Design review of the part built by this model. Coordinates are the model's own, in mm. Face numbers are marked on the shaded views. A direction names the side the tool comes from. Coordinates: 2 decimals unless noted, no trailing zeros. Write each loop counter-clockwise with the first axis right and the second up, starting at its lowest first coordinate (ties: lowest second). Pieces come first, ordered by that corner, then holes. Notation, with made-up numbers: M 72,20.5 L 76,20.5 A18 ccw 76,31.5 Z; hole C 67,-22 d1. An arc over 180 degrees is marked long. Write item = value, one per line.
```python
from build123d import *

# Parameters (mm, degrees)
BOSS_EXTRUDE1_DEPTH = 24
SKETCH1_4_W         = 12
SKETCH1_4_H         = 25
BOSS_EXTRUDE3_DEPTH = 60
BOSS_EXTRUDE5_DEPTH = 80
CUT_EXTRUDE4_DEPTH  = 104
BOSS_EXTRUDE6_DEPTH = 46
SKETCH5_W           = 44
SKETCH5_H           = 20
CUT_EXTRUDE5_DEPTH  = 46


with BuildPart() as part:
    # Sketch1 → Boss-Extrude1 (new body)
    with BuildSketch(Plane(origin=(0, 0, 0), x_dir=(1, 0, 0), z_dir=(0, 1, 0))):
        with BuildLine():
            Line((-50.214859888, 8.694484644), (-50.214859888, -16.305515356))
            Line((-50.214859888, -16.305515356), (-42.214859888, -16.305515356))
            ThreePointArc((-42.214859888, -16.305515356), (-12.214859888, 13.694484644), (17.785140112, -16.305515356))
            Line((17.785140112, -16.305515356), (25.785140112, -16.305515356))
            Line((25.785140112, -16.305515356), (25.785140112, 8.694484644))
            Line((25.785140112, 8.694484644), (25.785140112, 16.694484644))
            Line((25.785140112, 16.694484644), (-50.214859888, 16.694484644))
            Line((-50.214859888, 16.694484644), (-50.214859888, 8.694484644))
        make_face()
    extrude(amount=BOSS_EXTRUDE1_DEPTH)

    # Sketch1<4> → Boss-Extrude3 (add)
    with BuildSketch(Plane(origin=(0, 0, 0), x_dir=(1, 0, 0), z_dir=(0, 1, 0))):
        with Locations((-56.214859888, -3.805515356)):
            Rectangle(SKETCH1_4_W, SKETCH1_4_H)
        with Locations((31.785140112, -3.805515356)):
            Rectangle(SKETCH1_4_W, SKETCH1_4_H)
    extrude(amount=BOSS_EXTRUDE3_DEPTH)

    # Sketch1<7> → Boss-Extrude5 (add)
    with BuildSketch(Plane(origin=(0, 0, 0), x_dir=(1, 0, 0), z_dir=(0, 1, 0))):
        Polygon((-62.214859888, 28.694484644), (-62.214859888, 8.694484644), (-50.214859888, 8.694484644), (-50.214859888, 16.694484644), (25.785140112, 16.694484644), (25.785140112, 8.694484644), (37.785140112, 8.694484644), (37.785140112, 28.694484644), align=None)
    extrude(amount=BOSS_EXTRUDE5_DEPTH)

    # Sketch3 → Cut-Extrude4 (cut)
    with BuildSketch(Plane.ZY.offset(62.214859888)):
        Polygon((16.305515356, 24), (-8.694484644, 60), (16.305515356, 60), align=None)
    extrude(amount=-CUT_EXTRUDE4_DEPTH, mode=Mode.SUBTRACT)

    # Sketch1<8> → Boss-Extrude6 (add)
    with BuildSketch(Plane(origin=(0, 0, 0), x_dir=(1, 0, 0), z_dir=(0, 1, 0))):
        with BuildLine():
            ThreePointArc((17.785140112, -16.305515356), (-12.214859888, 13.694484644), (-42.214859888, -16.305515356))
            Line((-42.214859888, -16.305515356), (-30.214859888, -16.305515356))
            ThreePointArc((-30.214859888, -16.305515356), (-12.214859888, 1.694484644), (5.785140112, -16.305515356))
            Line((5.785140112, -16.305515356), (17.785140112, -16.305515356))
        make_face()
    extrude(amount=BOSS_EXTRUDE6_DEPTH)

    # Sketch5 → Cut-Extrude5 (cut)
    with BuildSketch(Plane.XY.offset(-16.694484644)):
        with Locations((-12.214859888, 58)):
            Rectangle(SKETCH5_W, SKETCH5_H)
    extrude(amount=-CUT_EXTRUDE5_DEPTH, mode=Mode.SUBTRACT)


solid = part.part
```
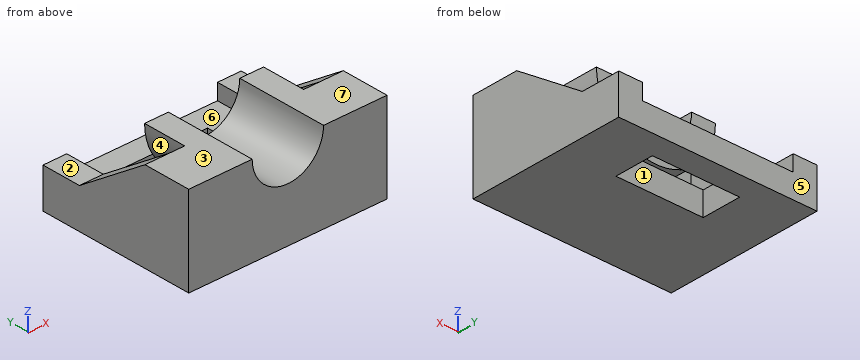
Q1. Consider section B-B, the plane z = 1.5. State the section outline as (x, y) points, and give its area (3 significant figures).
Check result:
outline = M -62.21,0 L -22.45,0 L -22.45,46 L -38.31,46 L -38.31,24 L -50.21,24 L -50.21,45.32 L -62.21,45.32 Z; M -1.98,0 L 37.79,0 L 37.79,45.32 L 25.79,45.32 L 25.79,24 L 13.88,24 L 13.88,46 L -1.98,46 Z
area = 3,120 mm²
Q2. For P1, Ø24, axis at x = -15, z = 7, coming from the +Y side; P2, Ø4, axis at x = -44, z = 8.5, coming from the +Y side; P3, Ø9.5, axis at x = -59, y = 67.5, coming from the +Z side, all flat-tipped, find the tip position at first contact; note any pin that passes through.
Check result:
P1 = 46
P2 = 24
P3 = -8.69
Q3. Consider section A-A, the plane y = 65. State the section outline as (x, z) points, and give its area (3 significant figures).
Check result:
outline = M -62.21,-28.69 L -34.21,-28.69 L -34.21,-16.69 L -50.21,-16.69 L -50.21,-8.69 L -62.21,-8.69 Z; M 9.79,-28.69 L 37.79,-28.69 L 37.79,-8.69 L 25.79,-8.69 L 25.79,-16.69 L 9.79,-16.69 Z
area = 864 mm²
Q4. Machinability: for the marked faces 1, 2, 3 and 4, which of the approach directions +Z, -Z, +X, -X, +Y, -Y give a long, thin tool a straight path to every point of the face, cutting with its end or side? Answer none if there is none.
Check result:
face_1 = +Z, -Z
face_2 = +Z, +X, -X, +Y
face_3 = +Z, +X, -X, +Y, -Y
face_4 = +Y
Q5. Consider section C-C, the plane x = -27. State the section outline as (y, z) points.
Check result:
outline = M 0,-28.69 L 48,-28.69 L 48,-16.69 L 24,-16.69 L 24,-9.8 L 46,-9.8 L 46,6.04 L 0,6.04 Z; M 68,-28.69 L 80,-28.69 L 80,-16.69 L 68,-16.69 Z
Q6. Consider section D-D, the plane z = -25. State the section outline as (x, y) points.
Check result:
outline = M -62.21,0 L 37.79,0 L 37.79,80 L -62.21,80 Z; hole M -34.21,48 L 9.79,48 L 9.79,68 L -34.21,68 Z
Q7. Wall thickness on line 1 (X direction, y = 28, z = -5); line 2 (Y direction, x = -13.5, z = -24); line 3 (X direction, y = 49, z = -24): over which ranges is each line inside the solid? List them lowest first.
Check result:
line_1 = -62.21 to -50.21, -33.34 to 8.91, 25.79 to 37.79
line_2 = 0 to 48, 68 to 80
line_3 = -62.21 to -34.21, 9.79 to 37.79
Q8. The part is to be moulded in two halves that separate along Z. For the marked faces 5, 6 and 7, say which applies: +Z half, -Z half, draft (parallel to the pull), parting line (faces both ways), or undercut.
Check result:
face_5 = draft
face_6 = undercut
face_7 = +Z half
